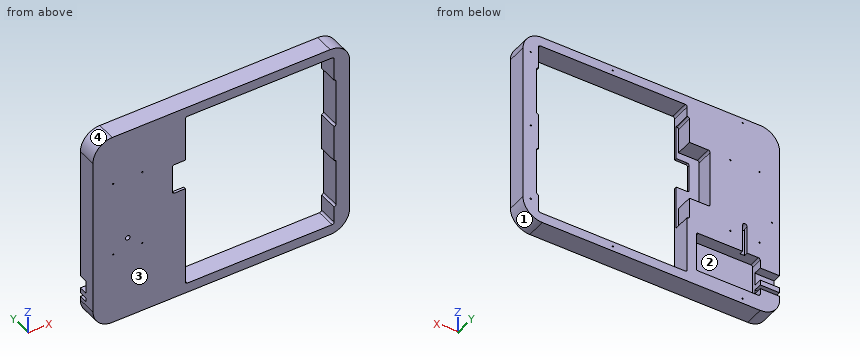
```python
from build123d import *

# Parameters (mm, degrees)
F0_W      = 397
F0_H      = 305
F1_DEPTH  = 30
F2_W      = 230
F2_H      = 275
F3_DEPTH  = 30
F4_R      = 3
F5_R      = 30
F6_W      = 26
F6_H      = 167
F7_DEPTH  = 3.5
F8_R      = 3
F10_W     = 32
F10_H     = 92
F11_DEPTH = 26
F12_R     = 3
F13_W     = 4
F13_H     = 47
F14_DEPTH = 20
F15_R     = 3
F16_W     = 30
F16_H     = 76.5
F17_DEPTH = 3
F18_R     = 2.99999
F19_R     = 3.5
F20_DEPTH = 30
F21_W     = 99
F21_H     = 62
F22_DEPTH = 18
F23_R     = 3
F25_DEPTH = 6
F26_W     = 13
F26_H     = 20
F26_H_2   = 6
F27_DEPTH = 30
F28_R     = 1
F29_DEPTH = 30
F31_DEPTH = 20


# Not quite as in the source:
# - a fillet or chamfer is up to 0.001 mm smaller than in the source, because OpenCascade refuses the exact size
# - a feature names something its author has since deleted; it is built from what else it names


with BuildPart() as f1:
    # F0 (on Front) → F1 (new body)
    with BuildSketch(Plane.XZ):
        with Locations((0, 5)):
            Rectangle(F0_W, F0_H)
    extrude(amount=F1_DEPTH)

    # F2 (on face) → F3 (cut, through all)
    with BuildSketch(Plane.XZ.offset(30)):
        with Locations((59.5, 5)):
            Rectangle(F2_W, F2_H)
    extrude(amount=-F3_DEPTH, mode=Mode.SUBTRACT)

    # F4
    f4_edges = [f1.edges().sort_by_distance(p)[0] for p in [
        (-55.5, -15, 142.5),
        (174.5, -15, 142.5),
        (174.5, -15, -132.5),
        (-55.5, -15, -132.5),
    ]]
    fillet(f4_edges, radius=F4_R)

    # F5
    f5_edges = [f1.edges().sort_by_distance(p)[0] for p in [
        (-198.5, -15, -147.5),
        (-198.5, -15, 157.5),
        (198.5, -15, 157.5),
        (198.5, -15, -147.5),
    ]]
    fillet(f5_edges, radius=F5_R)

    # F6 (on face) → F7 (cut)
    with BuildSketch(Plane.YZ.offset(-55.5)):
        with Locations((-13, 40.5)):
            Rectangle(F6_W, F6_H)
    extrude(amount=-F7_DEPTH, mode=Mode.SUBTRACT)

    # F8
    f8_edges = [f1.edges().sort_by_distance(p)[0] for p in [
        (-59, -13, -43),
        (-59, -13, 124),
    ]]
    fillet(f8_edges, radius=F8_R)

    # F10 (on face) → F11 (cut)
    with BuildSketch(Plane(origin=(0, 0, 0), x_dir=(-1, 0, 0), z_dir=(0, 1, 0))):
        with Locations((75, 36.5)):
            Rectangle(F10_W, F10_H)
    extrude(amount=-F11_DEPTH, mode=Mode.SUBTRACT)

    # F12
    f12_edges = [f1.edges().sort_by_distance(p)[0] for p in [
        (-91, -13, -9.5),
        (-91, -13, 82.5),
    ]]
    fillet(f12_edges, radius=F12_R)

    # F13 (on face) → F14 (cut)
    with BuildSketch(Plane.YZ.offset(-55.5)):
        with Locations((-28, 48)):
            Rectangle(F13_W, F13_H)
    extrude(amount=-F14_DEPTH, mode=Mode.SUBTRACT)

    # F15
    f15_edges = [f1.edges().sort_by_distance(p)[0] for p in [
        (-75.5, -28, 24.5),
        (-75.5, -28, 71.5),
    ]]
    fillet(f15_edges, radius=F15_R)

    # F16 (on face) → F17 (cut)
    with BuildSketch(Plane(origin=(174.5, 0, 0), x_dir=(0, -1, 0), z_dir=(-1, 0, 0))):
        with Locations((15, -66.25)):
            Rectangle(F16_W, F16_H)
        with Locations((15, 66.25)):
            Rectangle(F16_W, F16_H)
    extrude(amount=-F17_DEPTH, mode=Mode.SUBTRACT)

    # F18 (radius 3 in the source; OpenCascade refuses exactly that, so slightly less here)
    f18_edges = [f1.edges().sort_by_distance(p)[0] for p in [
        (177.5, -15, -104.5),
        (177.5, -15, 28),
        (177.5, -15, 104.5),
        (177.5, -15, -28),
    ]]
    fillet(f18_edges, radius=F18_R)

    # F19 (on face) → F20 (cut)
    with BuildSketch(Plane.XZ.offset(30)):
        with Locations((-144.75, -18.25)):
            Circle(F19_R)
    extrude(amount=-F20_DEPTH, mode=Mode.SUBTRACT)

    # F21 (on face) → F22 (cut)
    with BuildSketch(Plane(origin=(0, 0, 0), x_dir=(-1, 0, 0), z_dir=(0, 1, 0))):
        with Locations((119, -92.75)):
            Rectangle(F21_W, F21_H)
    extrude(amount=-F22_DEPTH, mode=Mode.SUBTRACT)

    # F23
    f23_edges = [f1.edges().sort_by_distance(p)[0] for p in [
        (-168.5, -9, -123.75),
        (-69.5, -9, -123.75),
        (-69.5, -9, -61.75),
        (-168.5, -9, -61.75),
    ]]
    fillet(f23_edges, radius=F23_R)

    # F24 (on face) → F25 (cut)
    with BuildSketch(Plane(origin=(0, 0, 0), x_dir=(-1, 0, 0), z_dir=(0, 1, 0))):
        with BuildLine():
            ThreePointArc((148.25, -18.25), (144.75, -21.75), (141.25, -18.25))
            Line((141.25, -18.25), (141.25, -61.75))
            Line((141.25, -61.75), (148.25, -61.75))
            Line((148.25, -61.75), (148.25, -18.25))
        make_face()
    extrude(amount=-F25_DEPTH, mode=Mode.SUBTRACT)

    # F26 (on face) → F27 (cut)
    with BuildSketch(Plane(origin=(-198.5, 0, 0), x_dir=(0, -1, 0), z_dir=(-1, 0, 0))):
        with Locations((6.5, -87.5)):
            Rectangle(F26_W, F26_H)
        with Locations((6.5, -108.5)):
            Rectangle(F26_W, F26_H_2)
    extrude(amount=-F27_DEPTH, mode=Mode.SUBTRACT)

    # F28 (on face) → F29 (cut)
    with BuildSketch(Plane.XZ.offset(30)):
        with Locations((-167.25, 80.35)):
            Circle(F28_R)
        with Locations((-167.25, -36.25)):
            Circle(F28_R)
        with Locations((-122.25, -36.25)):
            Circle(F28_R)
        with Locations((-122.25, 80.35)):
            Circle(F28_R)
    extrude(amount=-F29_DEPTH, mode=Mode.SUBTRACT)

    # F30 (on face) → F31 (cut)
    with BuildSketch(Plane(origin=(0, 0, 0), x_dir=(-1, 0, 0), z_dir=(0, 1, 0))):
        with BuildLine():
            Line((-186.5, 125), (-186.5, 127))
            ThreePointArc((-186.5, 127), (-187.5, 126), (-186.5, 125))
        make_face()
        with BuildLine():
            ThreePointArc((-185.5, 126), (-185.7928932188, 126.7071067812), (-186.5, 127))
            Line((-186.5, 127), (-186.5, 125))
            ThreePointArc((-186.5, 125), (-185.7928932188, 125.2928932188), (-185.5, 126))
        make_face()
        with BuildLine():
            ThreePointArc((-60.5, 150), (-59.5, 149), (-58.5, 150))
            Line((-58.5, 150), (-60.5, 150))
        make_face()
        with BuildLine():
            Line((-60.5, 150), (-58.5, 150))
            ThreePointArc((-58.5, 150), (-59.5, 151), (-60.5, 150))
        make_face()
        with BuildLine():
            Line((140.25, 150), (142.25, 150))
            ThreePointArc((142.25, 150), (141.25, 151), (140.25, 150))
        make_face()
        with BuildLine():
            ThreePointArc((140.25, 150), (141.25, 149), (142.25, 150))
            Line((142.25, 150), (140.25, 150))
        make_face()
        with BuildLine():
            ThreePointArc((187.5, 5), (187.2071067812, 5.7071067812), (186.5, 6))
            Line((186.5, 6), (186.5, 4))
            ThreePointArc((186.5, 4), (187.2071067812, 4.2928932188), (187.5, 5))
        make_face()
        with BuildLine():
            Line((186.5, 4), (186.5, 6))
            ThreePointArc((186.5, 6), (185.5, 5), (186.5, 4))
        make_face()
        with BuildLine():
            Line((140.25, -140), (142.25, -140))
            ThreePointArc((142.25, -140), (141.25, -139), (140.25, -140))
        make_face()
        with BuildLine():
            ThreePointArc((140.25, -140), (141.25, -141), (142.25, -140))
            Line((142.25, -140), (140.25, -140))
        make_face()
        with BuildLine():
            Line((-60.5, -140), (-58.5, -140))
            ThreePointArc((-58.5, -140), (-59.5, -139), (-60.5, -140))
        make_face()
        with BuildLine():
            ThreePointArc((-60.5, -140), (-59.5, -141), (-58.5, -140))
            Line((-58.5, -140), (-60.5, -140))
        make_face()
        with BuildLine():
            ThreePointArc((-185.5, -116), (-185.7928932188, -115.2928932188), (-186.5, -115))
            Line((-186.5, -115), (-186.5, -117))
            ThreePointArc((-186.5, -117), (-185.7928932188, -116.7071067812), (-185.5, -116))
        make_face()
        with BuildLine():
            Line((-186.5, -117), (-186.5, -115))
            ThreePointArc((-186.5, -115), (-187.5, -116), (-186.5, -117))
        make_face()
        with BuildLine():
            Line((-186.5, 4), (-186.5, 6))
            ThreePointArc((-186.5, 6), (-187.5, 5), (-186.5, 4))
        make_face()
        with BuildLine():
            ThreePointArc((-185.5, 5), (-185.7928932188, 5.7071067812), (-186.5, 6))
            Line((-186.5, 6), (-186.5, 4))
            ThreePointArc((-186.5, 4), (-185.7928932188, 4.2928932188), (-185.5, 5))
        make_face()
    extrude(amount=-F31_DEPTH, mode=Mode.SUBTRACT)


solid = f1.part
```
Model file for the job. Use its own axes, mm. Face numbers are marked on the shaded views. Coordinates: 2 decimals unless noted, no trailing zeros. Loops run counter-clockwise (first coordinate to the right, second up) from the corner with the lowest first, then second, coordinate; pieces in that order, holes last. Notation, with made-up numbers: (-3, -24) - (30, -24) arc R23 ccw to (30, 7) - close; hole circle Ø7 at (55, -14). An arc over 180 degrees is marked (long way). Answer as a JSON object with one key per item and string values. Group by question number.
(1) Two-plate mould, pull along Z, no slides. Class the marked faces 1, 2, 3 and 4: released by +Z, released by -Z, zero draft, split by the parting line, or undercut.
(2) Cut at A-A (z = 49). Give the cut face in (x, y).
(3) Flat gauge pins, fed straight in: pin 1 (4 mm diameter, centred on x = -176, y = -4, fed in from -Z); pin 2 (14.5 mm diameter, centred on x = -179.5, y = -5.5, fed in from +Z); pin 3 (5.5 mm diameter, centred on x = -144.75, z = -18.25, fed in from +Y); pin 4 (1.6 mm diameter, centred on x = 59.5, z = -140, fed in from +Y). Where does each tip first touch, or does it go through?
(4) Cut at C-C (z = 134.5). Give the cut face in (x, y), then the cut area to 3 significant figures.
(5) Cut at B-B (x = 133.5). Give the cut face in (y, z), then the cut area to 3 significant figures.
(6) Probe line 1 along Z through (x, y) = (59.5, -8.25); line 2 along Z through (x, y) = (-122.25, -18.5); line 3 along X through (y, z) = (-9.75, -60). List the from-to ranges inside material, lowest first.
Geometry says:
{
 "1": {"face 1": "released by -Z", "face 2": "undercut", "face 3": "zero draft", "face 4": "released by +Z"},
 "2": {"outline": "(-198.5, -30) - (-75.5, -30) - (-75.5, -26) - (-91, -26) - (-91, 0) - (-198.5, 0) - close; (177.5, -30) - (198.5, -30) - (198.5, 0) - (177.5, 0) - close"},
 "3": {"pin 1": "stops at z = -146.99", "pin 2": "stops at z = 157.26", "pin 3": "passes through", "pin 4": "stops at y = -20"},
 "4": {"outline": "(-197.67, -30) - (-55.5, -30) - (-55.5, 0) - (-197.67, 0) - close; (174.5, -30) - (197.67, -30) - (197.67, 0) - (174.5, 0) - close", "area": "4,960 mm^2"},
 "5": {"outline": "(-30, -147.5) - (0, -147.5) - (0, -132.5) - (-30, -132.5) - close; (-30, 142.5) - (0, 142.5) - (0, 157.5) - (-30, 157.5) - close", "area": "900 mm^2"},
 "6": {"line 1": "z = -147.5 to -141, -139 to -132.5, 142.5 to 149, 151 to 157.5", "line 2": "z = -147.5 to -37.25, -35.25 to 79.35, 81.35 to 157.5", "line 3": "x = -198.5 to -55.5, 177.5 to 198.5"}
}
